Design review of the part shown in the three views and the two pictorial views. Dimensions are in mm from the part's minimum x, y and z. A direction names the side the tool comes from. Coordinates: 2 decimals unless noted, no trailing zeros. Loops run counter-clockwise (first coordinate to the right, second up) from the corner with the lowest first, then second, coordinate; pieces in that order, holes last. Notation, with made-up numbers: (-20, -14.75) - (1, -14.75) arc R33 ccw to (1, 13.25) - close; hole circle Ø5 at (9.25, 88). An arc over 180 degrees is marked (long way). One line per question, with ' | ' between items.
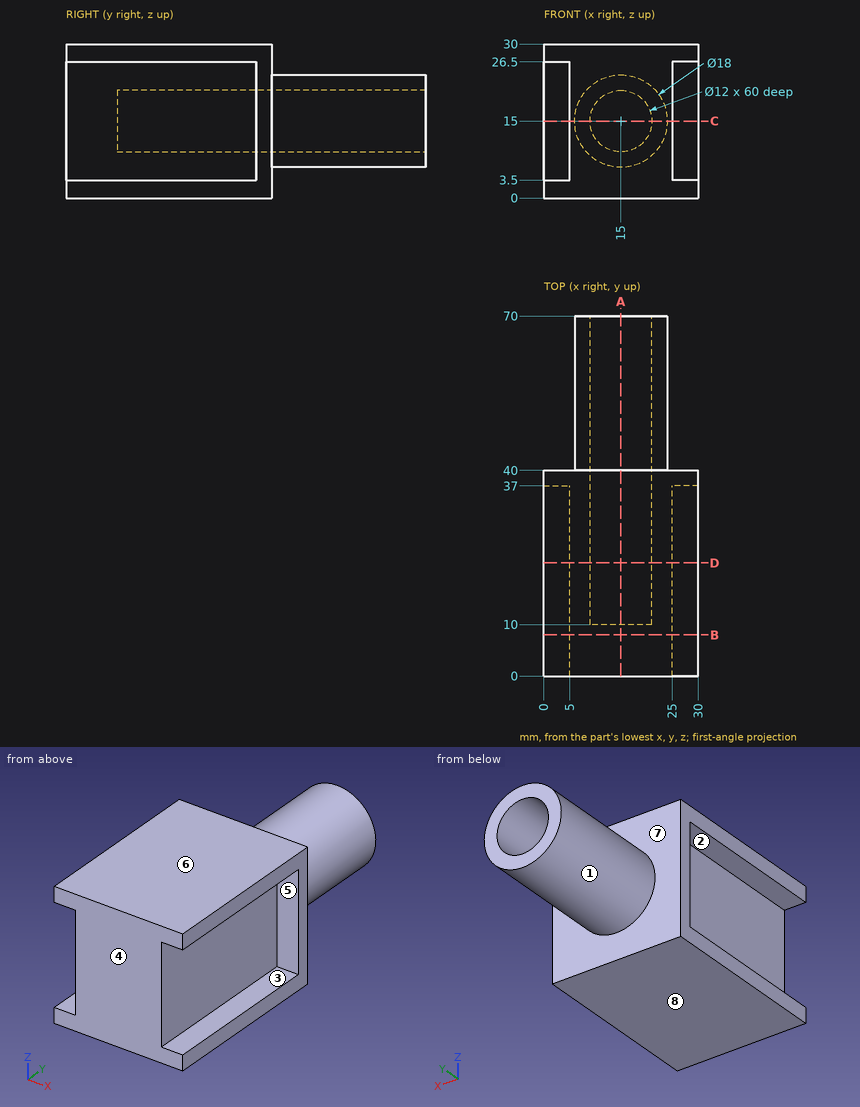
Q1. Draft analysis for pull direction Z (two halves, no side actions). For the marked faces 5, 6, 7 and 8, state which applies: +Z half, -Z half, draft (parallel to the pull), parting line (faces both ways), or undercut.
Returned:
face 5: undercut | face 6: +Z half | face 7: draft | face 8: -Z half
Q2. Tool access review of the marked faces 1, 2, 3 and 4: name each direction out of +Z, -Z, +X, -X, +Y, -Y from which nothing blocks a thin tool from reaching the whole face with its end or side.
Returned:
face 1: +Y | face 2: -X, -Y | face 3: +X, -Y | face 4: +Z, -Z, +X, -X, -Y
Q3. Take a section at A-A (x = 15). Give the boundary of the cut face in (y, z).
Returned:
outline: (0, 0) - (40, 0) - (40, 6) - (70, 6) - (70, 9) - (10, 9) - (10, 21) - (70, 21) - (70, 24) - (40, 24) - (40, 30) - (0, 30) - close
Q4. For pin 1 (1.5 mm diameter, centred on x = 3.5, z = 12, fed in from -Y); pin 2 (6 mm diameter, centred on x = 17, z = 15, fed in from +Y); pin 3 (5.5 mm diameter, centred on x = 2, y = 25, fed in from -Z); pin 4 (1 mm diameter, centred on y = 20, z = 8, fed in from -X), all flat-tipped, find the tip position at first contact; note any pin that passes through.
Returned:
pin 1: stops at y = 37 | pin 2: stops at y = 10 | pin 3: stops at z = 0 | pin 4: stops at x = 5
Q5. Take a section at D-D (y = 22). Give the boundary of the cut face in (x, z), plus the area to 3 significant figures.
Returned:
outline: (0, 0) - (30, 0) - (30, 3.5) - (25, 3.5) - (25, 26.5) - (30, 26.5) - (30, 30) - (0, 30) - (0, 26.5) - (5, 26.5) - (5, 3.5) - (0, 3.5) - close; hole circle Ø12 at (15, 15) | area: 557 mm²
Q6. Take a section at C-C (z = 15). Give the boundary of the cut face in (x, y).
Returned:
outline: (0, 37) - (5, 37) - (5, 0) - (25, 0) - (25, 37) - (30, 37) - (30, 40) - (24, 40) - (24, 70) - (21, 70) - (21, 10) - (9, 10) - (9, 70) - (6, 70) - (6, 40) - (0, 40) - close
Q7. Take a section at B-B (y = 8). Give the boundary of the cut face in (x, z).
Returned:
outline: (0, 0) - (30, 0) - (30, 3.5) - (25, 3.5) - (25, 26.5) - (30, 26.5) - (30, 30) - (0, 30) - (0, 26.5) - (5, 26.5) - (5, 3.5) - (0, 3.5) - close
Q8. To check wall thickness, follow line 1 along X through (y, z) = (24, 15); line 2 along X through (y, z) = (55.5, 15); line 3 along Z through (x, y) = (14.75, 16). State the ranges of each line that lie inside material, in increasing order.
Returned:
line 1: x = 5 to 9, 21 to 25 | line 2: x = 6 to 9, 21 to 24 | line 3: z = 0 to 9.01, 20.99 to 30
